Geometry: final body of the model. Coordinates: model frame, mm. Face numbers are marked on the shaded views. A direction names the side the tool comes from. Round coordinates to 2 decimals unless told otherwise and drop trailing zeros. Order: outer loops, then holes, each group sorted by start corner. A loop starts at its lowest first (then second) coordinate and runs counter-clockwise, first axis right, second up. Notation, with made-up numbers: M 11,79.5 L 19,79.5 A11 ccw 19,84.5 Z; hole C -35.75,85 d11. An arc over 180 degrees is marked long. Return JSON: item names as keys, results as strings. Group by question number.
Q1. Cut plane B-B on z = -1.85. Output: boundary loops of the cut face in (x, y), and give its area (3 significant figures).
Q2. Mould query, pull axis X, two halves, no side actions, for the marked faces 1, 2 and 3. Classes: released by +X, released by -X, zero draft, split by the parting line, or undercut.
Q3. Cut plane C-C on y = 4.5. Output: boundary loops of the cut face in (x, z).
Q4. Ray query, probe 1 along Z at (x, y) = (0.25, -2); probe 2 along Z at (x, y) = (1.75, 4.25); probe 3 along X at (y, z) = (0, 2.05). Return the intervals inside material, ascending.
Q5. Access query for the marked faces 4, 5 and 6. Directions: +Z, -Z, +X, -X, +Y, -Y. A direction counts if a zero-diameter tool reaches every point of the face in a straight line with its end or side. Return the directions, or none.
Q6. Cut plane D-D on z = 1.35. Output: boundary loops of the cut face in (x, y), and give its area (3 significant figures).
Q7. Contact query for flat-ended pins moving along their axis: pin 1 (1.5 mm diameter, centred on x = -3.5, y = -3.5, fed in from -Z); pin 2 (5 mm diameter, centred on x = -0.5, y = 0.5, fed in from +Z); pin 3 (1.5 mm diameter, centred on x = 1.5, z = -2, fed in from -Y). Output: stop coordinate, or through.
Autodesk Inventor part; units mm, degrees
ref_plane "YZ Plane" through (0, 0, 0) normal (1, 0, 0) x (0, 1, 0)
ref_plane "XZ Plane" through (0, 0, 0) normal (0, 1, 0) x (-1, 0, 0)
ref_plane "XY Plane" through (0, 0, 0) normal (0, 0, 1) x (1, 0, 0)
sketch "Sketch1" plane through (0, 0, 0) normal (0, 0, 1) x (1, 0, 0)
  circle A0 centre (0, 0) radius 3
  circle A1 centre (0, 0) radius 3
  point P0 (0, 0)
  dimension "d0" = 6
extrude "Extrusion1" add sketch "Sketch1" against normal blind 3
sketch "Sketch2" plane through (0, 0, 0) normal (0, 0, 1) x (1, 0, 0)
  circle A0 centre (0, 0) radius 3
  circle A1 centre (0, 0) radius 11
  circle A2 centre (0, 0) radius 3
  circle A3 centre (8, 0) radius 1.5
  circle A4 centre (0, 8) radius 1.5
  circle A5 centre (-8, 0) radius 1.5
  circle A6 centre (0, -8) radius 1.5
  circle A7 centre (0, 0) radius 5
  point P0 (0, 0)
  dimension "d3" = 10
extrude "Extrusion2" add sketch "Sketch2" along normal blind 2 contours A0 | A7
sketch "Sketch3" plane through (0, 0, 2) normal (0, 0, 1) x (1, 0, 0)
  circle A0 centre (0, 0) radius 5
  circle A1 centre (0, 0) radius 3
  circle A2 centre (0, 0) radius 3
  point P0 (0, 0)
  dimension "d6" = 6
extrude "Extrusion3" add sketch "Sketch3" along normal blind 1
chamfer "Chamfer1" distance 1 angle 45 1 edges at (-3, 0, 3)
thicken "Thicken1" operation add thickness 0.05 both sides no extend neighbours yes toward (-0.9967573, 0.0804666, 0) faces at (2.9903, -0.2414, -2)
chamfer "Chamfer2" distance 0.5 angle 45 1 edges at (-2.95, 0, -3)
properties part number "encoder_ma_holder"
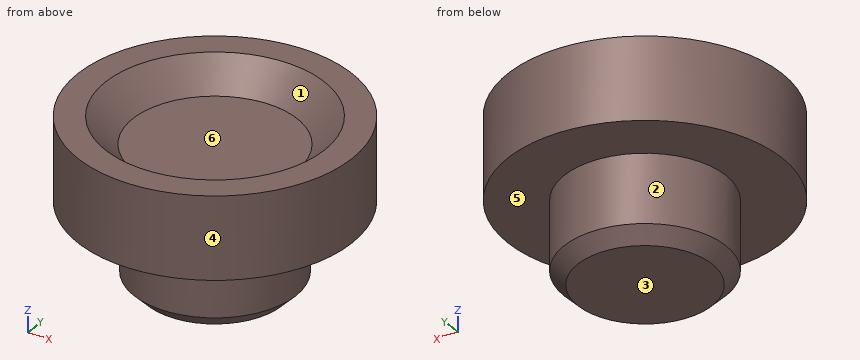
Result sheet:
{
 "1": {"outline": "C 0,0 d5.9", "area": "27.3 mm²"},
 "2": {"face 1": "undercut", "face 2": "split by the parting line", "face 3": "zero draft"},
 "3": {"outline": "M -2.18,0 L 2.18,0 L 2.18,3 L -2.18,3 Z"},
 "4": {"probe 1": "z = -3 to 2", "probe 2": "z = 0 to 3", "probe 3": "x = -5 to -3.05, 3.05 to 5"},
 "5": {"face 4": "+Z, -Z", "face 5": "-Z", "face 6": "+Z"},
 "6": {"outline": "C 0,0 d10", "area": "78.5 mm²"},
 "7": {"pin 1": "stops at z = 0", "pin 2": "stops at z = 2.21", "pin 3": "stops at y = -2.85"}
}
